from build123d import *

# Parameters (mm, degrees)
F0_R        = 20
F1_DEPTH    = 15
F0_R_2      = 10
F2_DEPTH    = 7.5
F3_T1_DEPTH = 7.5
F3_T3_DEPTH = 7.5


# Not quite as in the source:
# - a fillet or chamfer that OpenCascade refuses, or shapes differently, is made with other operations: its cross-section is extruded or revolved along the edge and cut away or added


with BuildPart() as f1:
    # F0 (on Front) → F1 (new body, symmetric)
    with BuildSketch(Plane.XZ):
        with BuildLine():
            ThreePointArc((-24.128180818, -21.7733986877), (11.6637070311, -30.3349293438), (32.5, 0))
            ThreePointArc((32.5, 0), (30.7312117377, 10.5755673669), (25.6173769149, 20))
            ThreePointArc((25.6173769149, 20), (-20.899967362, 24.8885789925), (-24.128180818, -21.7733986877))
        make_face()
        Circle(F0_R, mode=Mode.SUBTRACT)
    extrude(amount=F1_DEPTH, both=True)



with BuildPart() as f1b:
    # F0 (on Front) → F1, piece 2 (new body, symmetric)
    with BuildSketch(Plane.XZ):
        with BuildLine():
            ThreePointArc((152.5, 0), (130.5755673669, 30.7312117377), (94.3826230851, 20))
            ThreePointArc((94.3826230851, 20), (99.100032638, -24.8885789925), (144.128180818, -21.7733986877))
            ThreePointArc((144.128180818, -21.7733986877), (150.3349293438, -11.6637070311), (152.5, 0))
        make_face()
        with Locations((120, 0)):
            Circle(F0_R, mode=Mode.SUBTRACT)
    extrude(amount=F1_DEPTH, both=True)


with BuildPart() as f1_1:
    add(f1.part)

    add(f1b.part)  # F2 merges F1b
    # F0 (on Front) → F2 (join, symmetric)
    with BuildSketch(Plane.XZ):
        with BuildLine():
            ThreePointArc((25.6173769149, 20), (30.7312117377, 10.5755673669), (32.5, 0))
            ThreePointArc((32.5, 0), (11.6637070311, -30.3349293438), (-24.128180818, -21.7733986877))
            Line((-24.128180818, -21.7733986877), (52.5759443637, -106.773036476))
            ThreePointArc((52.5759443637, -106.773036476), (60, -110.0735291875), (67.4240556363, -106.773036476))
            Line((67.4240556363, -106.773036476), (144.128180818, -21.7733986877))
            ThreePointArc((144.128180818, -21.7733986877), (99.100032638, -24.8885789925), (94.3826230851, 20))
            Line((94.3826230851, 20), (25.6173769149, 20))
        make_face()
        with Locations((60, -90.0735291875)):
            Circle(F0_R_2, mode=Mode.SUBTRACT)
    extrude(amount=F2_DEPTH, both=True)

    # F3: fillet of radius 15 on 4 edges, made by hand

    # F3_s2 → F3_t1 (join)
    with BuildSketch(Plane.XZ.offset(-7.5)):
        with BuildLine():
            ThreePointArc((32.1130814467, 20), (26.6720095708, 21.0216332556), (21.9721083582, 23.9473684211))
            ThreePointArc((21.9721083582, 23.9473684211), (23.8764571598, 22.0491449607), (25.6173769149, 20))
            Line((25.6173769149, 20), (32.1130814467, 20))
        make_face()
        with BuildLine():
            ThreePointArc((98.0278916418, 23.9473684211), (93.3279904292, 21.0216332556), (87.8869185533, 20))
            Line((87.8869185533, 20), (94.3826230851, 20))
            ThreePointArc((94.3826230851, 20), (96.1235428402, 22.0491449607), (98.0278916418, 23.9473684211))
        make_face()
    extrude(amount=F3_T1_DEPTH)

    # F3_s4 → F3_t3 (join)
    with BuildSketch(Plane.XZ):
        with BuildLine():
            ThreePointArc((32.1130814467, 20), (26.6720095708, 21.0216332556), (21.9721083582, 23.9473684211))
            ThreePointArc((21.9721083582, 23.9473684211), (23.8764571598, 22.0491449607), (25.6173769149, 20))
            Line((25.6173769149, 20), (32.1130814467, 20))
        make_face()
        with BuildLine():
            ThreePointArc((87.8869185533, 20), (93.3279904292, 21.0216332556), (98.0278916418, 23.9473684211))
            ThreePointArc((98.0278916418, 23.9473684211), (96.1235428402, 22.0491449607), (94.3826230851, 20))
            Line((94.3826230851, 20), (87.8869185533, 20))
        make_face()
    extrude(amount=F3_T3_DEPTH)


solid = f1_1.part
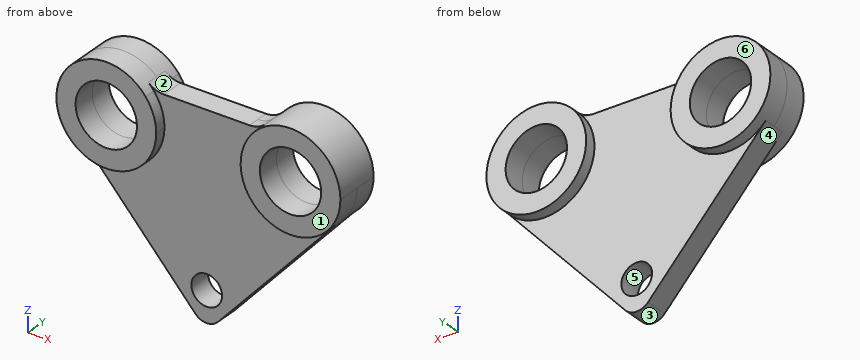
Build history of the part. All positions in model axes, mm. Face numbers are marked on the shaded views. A direction names the side the tool comes from. Give positions to 0.01 mm unless a question says otherwise; leave off trailing zeros. Loops run counter-clockwise (first coordinate to the right, second up) from the corner with the lowest first, then second, coordinate; pieces in that order, holes last. Notation, with made-up numbers: (-9, 34) -> (33, 34) arc R25 ccw to (33, 57) -> close; hole circle Ø3 at (38, 29.5). An arc over 180 degrees is marked (long way). Answer in a Markdown table with one row per item.
Item 1: Slice it at B-B on x = -12. Write the cut outline in (y, z).
Findings below:
| item | result |
|---|---|
| outline | (-15, -30.2) -> (-7.5, -30.2) -> (-7.5, -35.21) -> (7.5, -35.21) -> (7.5, -30.2) -> (15, -30.2) -> (15, -16) -> (-15, -16) -> close; (-15, 16) -> (15, 16) -> (15, 30.2) -> (-15, 30.2) -> close |
Item 2: Mould opens along X. For the marked faces 3, 4, 5 and 6 say: pulls with the +X half, pulls with the -X half, needs draft (parallel to the pull), parting line crosses it, or undercut.
Findings below:
| item | result |
|---|---|
| face 3 | parting line crosses it |
| face 4 | pulls with the -X half |
| face 5 | undercut |
| face 6 | needs draft |
Item 3: Slice it at D-D on x = 136.5. Write the cut outline in (y, z).
Findings below:
| item | result |
|---|---|
| outline | (-15, -28) -> (-7.5, -28) -> (-7.5, -30.23) -> (7.5, -30.23) -> (7.5, -28) -> (15, -28) -> (15, -11.3) -> (-15, -11.3) -> close; (-15, 11.3) -> (15, 11.3) -> (15, 28) -> (-15, 28) -> close |
Item 4: Probe line 1 along Z through (x, y) = (60, 2.25); line 2 along Z through (x, y) = (120, 9.5); line 3 along X through (y, z) = (-13.25, -14). List the from-to ranges inside material, lowest first. Write a range as [from, to].
Findings below:
| item | result |
|---|---|
| line 1 | z = [-110.07, -100.07], [-80.07, 20] |
| line 2 | z = [-32.5, -20], [20, 32.5] |
| line 3 | x = [-29.33, -14.28], [14.28, 29.33], [90.67, 105.72], [134.28, 149.33] |
Item 5: Tool access for the marked faces 1 and 2: list every direction of +Z, -Z, +X, -X, +Y, -Y with a clear straight run to the whole face (end or side of a thin tool).
Findings below:
| item | result |
|---|---|
| face 1 | +Z, -Z, +X, -X, -Y |
| face 2 | +Z, +Y, -Y |
Item 6: Flat gauge pins, fed straight in: P1, Ø3, axis at x = 23.5, y = 11, coming from the -Z side; P2, Ø6, axis at x = 16, y = 2, coming from the -Z side; P3, Ø8, axis at x = -4.5, y = 2, coming from the +Z side. Where does each tip first touch, or does it go through?
Findings below:
| item | result |
|---|---|
| P1 | stops at z = -23.92 |
| P2 | stops at z = -69.57 |
| P3 | stops at z = 32.5 |
Item 7: Slice it at C-C on z = -9. Write the cut outline in (x, y).
Findings below:
| item | result |
|---|---|
| outline | (-31.23, -15) -> (-17.86, -15) -> (-17.86, 15) -> (-31.23, 15) -> close; (17.86, -15) -> (31.23, -15) -> (31.23, -7.5) -> (88.77, -7.5) -> (88.77, -15) -> (102.14, -15) -> (102.14, 15) -> (88.77, 15) -> (88.77, 7.5) -> (31.23, 7.5) -> (31.23, 15) -> (17.86, 15) -> close; (137.86, -15) -> (151.23, -15) -> (151.23, 15) -> (137.86, 15) -> close |
Item 8: Slice it at A-A on y = -13. Write the cut outline in (x, z).
Findings below:
| item | result |
|---|---|
| outline | circle Ø65 at (0, 0); circle Ø65 at (120, 0); hole circle Ø40 at (0, 0); hole circle Ø40 at (120, 0) |
